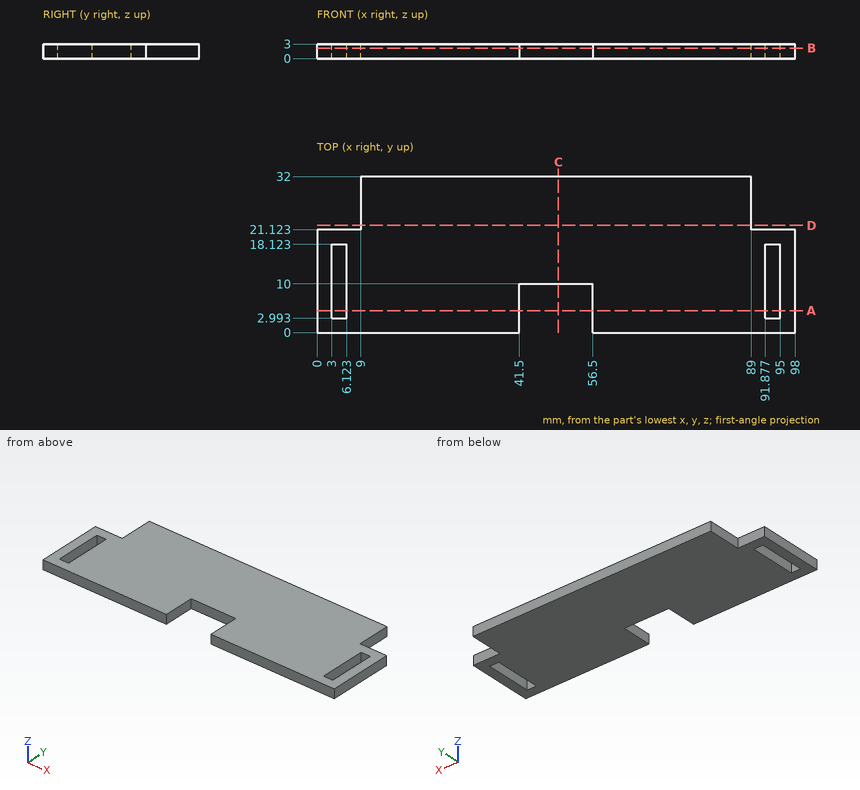
The figure shows three views and two pictorial views of one solid part (mm, origin at its lowest corner). Answer the questions. Give positions to 0.01 mm unless a question says otherwise; leave off trailing zeros. Order: outer loops, then holes, each group sorted by start corner. A loop starts at its lowest first (then second) coordinate and runs counter-clockwise, first axis right, second up. Notation, with made-up numbers: (0, 88) - (27, 88) arc R37 ccw to (27, 125) - close; hole circle Ø3 at (-35.75, 80). An arc over 180 degrees is marked (long way). Answer as CSV lines item,"result".
Q1. Each of these flat-tipped pins is pushed along its axis until it touches: pin 1 Ø1.5 at (y, z) = (28.5, 2) entering from +X; pin 2 Ø0.9 at (x, z) = (3, 1.5) entering from +Y; pin 3 Ø8 at (x, y) = (61.5, 7.5) entering from -Z; pin 4 Ø1.5 at (x, z) = (50, 1) entering from -Y. Where does it stop, or does it pass through?
Answer key:
pin 1,"stops at x = 89"
pin 2,"stops at y = 21.12"
pin 3,"stops at z = 0"
pin 4,"stops at y = 10"
Q2. A cutting plane is placed at D-D, the plane y = 22. Determine the outline of the cut face in (x, z).
Answer key:
outline,"(9, 0) - (89, 0) - (89, 3) - (9, 3) - close"
Q3. A cutting plane is placed at C-C, the plane x = 49.5. Determine the outline of the cut face in (y, z), and give its area (3 significant figures).
Answer key:
outline,"(10, 0) - (32, 0) - (32, 3) - (10, 3) - close"
area,"66.0 mm^2"
Q4. Straight lines are drawn through the part: L1, parallel to X at y = 9.5, z = 2.7; L2, parallel to Y at x = 48.5, z = 2.45; L3, parallel to X at y = 24, z = 1.9. For each, find the intervals that lie inside material, in ascending order.
Answer key:
L1,"x = 0 to 3, 6.12 to 41.5, 56.5 to 91.88, 95 to 98"
L2,"y = 10 to 32"
L3,"x = 9 to 89"
Q5. A cutting plane is placed at B-B, the plane z = 2.15. Determine the outline of the cut face in (x, y), and give its area (3 significant figures).
Answer key:
outline,"(0, 0) - (41.5, 0) - (41.5, 10) - (56.5, 10) - (56.5, 0) - (98, 0) - (98, 21.12) - (89, 21.12) - (89, 32) - (9, 32) - (9, 21.12) - (0, 21.12) - close; hole (3, 2.99) - (6.12, 2.99) - (6.12, 18.12) - (3, 18.12) - close; hole (91.88, 2.99) - (95, 2.99) - (95, 18.12) - (91.88, 18.12) - close"
area,"2,700 mm^2"
Q6. A cutting plane is placed at A-A, the plane y = 4.5. Determine the outline of the cut face in (x, z).
Answer key:
outline,"(0, 0) - (3, 0) - (3, 3) - (0, 3) - close; (6.12, 0) - (41.5, 0) - (41.5, 3) - (6.12, 3) - close; (56.5, 0) - (91.88, 0) - (91.88, 3) - (56.5, 3) - close; (95, 0) - (98, 0) - (98, 3) - (95, 3) - close"
